from build123d import *

# Parameters (mm, degrees)
SKETCH3_W               = 76.2
SKETCH3_H               = 158.75
BOSS_EXTRUDE1_DEPTH     = 53.975
SHELL1_T                = 6
FILLET1_R               = 5.334
FILLET2_R               = 6.35
CUT_EXTRUDE1_DEPTH      = 1.2446
FILLET3_R               = 0.254
FILLET4_R               = 0.127
SKETCH7_W               = 76.2
SKETCH7_H               = 2.5
BOSS_EXTRUDE2_DEPTH     = 53.975
BOSS_EXTRUDE3_DEPTH     = 29.972
SKETCH9_R               = 3.025
CUT_EXTRUDE2_DEPTH      = 9
MIRROR2_COPY_1_DEPTH    = 29.972
MIRROR2_COPY_2_SKETCH_R = 3.025
MIRROR2_COPY_2_DEPTH    = 9
BOSS_EXTRUDE4_DEPTH     = 29.972
SKETCH11_R              = 3.025
CUT_EXTRUDE3_DEPTH      = 9
BOSS_EXTRUDE5_DEPTH     = 29.972
SKETCH13_R              = 3.025
CUT_EXTRUDE4_DEPTH      = 9
SKETCH17_R              = 9.525
SKETCH17_R_2            = 6.35
CUT_EXTRUDE6_DEPTH      = 6
SKETCH18_R              = 14.2875
SKETCH18_R_2            = 10.795
CUT_EXTRUDE7_DEPTH      = 3


with BuildPart() as part:
    # Sketch3 → Boss-Extrude1 (new body)
    with BuildSketch(Plane.XY):
        with Locations((38.1, 79.375)):
            Rectangle(SKETCH3_W, SKETCH3_H)
    extrude(amount=BOSS_EXTRUDE1_DEPTH)

    # Shell1
    shell1_openings = [part.faces().sort_by_distance(p)[0] for p in [
        (38.1, 79.375, 0),
    ]]
    offset(amount=SHELL1_T, openings=shell1_openings, kind=Kind.INTERSECTION)

    # Fillet1
    # the kernel refuses this fillet: 5.334 mm, written as the material it adds along each edge
    with BuildSketch(Plane(origin=(0, 158.75, 0), x_dir=(1, 0, 0), z_dir=(0, 0, 1)), Plane(origin=(76.2, 0, 0), x_dir=(-1, 0, 0), z_dir=(0, 0, 1)), Plane(origin=(76.2, 158.75, 0), x_dir=(0, -1, 0), z_dir=(0, 0, 1))) as fillet1_piece_1:
        with BuildLine():
            CenterArc((FILLET1_R, -FILLET1_R), FILLET1_R, 90, 90)
            Line((0, -FILLET1_R), (0, 0))
            Line((0, 0), (FILLET1_R, 0))
        make_face()
    extrude(amount=53.975)
    with BuildSketch(Plane(origin=(0, 0, 0), x_dir=(1, 0, 0), z_dir=(0, 0, 1))) as fillet1_piece_2:
        with BuildLine():
            CenterArc((FILLET1_R, FILLET1_R), FILLET1_R, 180, 90)
            Line((0, FILLET1_R), (0, 0))
            Line((0, 0), (FILLET1_R, 0))
        make_face()
    extrude(amount=53.975)

    # Fillet2
    fillet2_edges = [part.edges().sort_by_distance(p)[0] for p in [
        (-6, 164.75, 29.9875),
        (82.2, 164.75, 29.9875),
        (82.2, -6, 29.9875),
        (-6, -6, 29.9875),
    ]]
    fillet(fillet2_edges, radius=FILLET2_R)

    # Sketch6 → Cut-Extrude1 (cut)
    with BuildSketch(Plane(origin=(0, 0, 0), x_dir=(-1, 0, 0), z_dir=(0, 0, -1))):
        with BuildLine():
            Line((-5.334, 163.0327), (-70.866, 163.0327))
            ThreePointArc((-70.866, 163.0327), (-77.666033783, 160.216033783), (-80.4827, 153.416))
            Line((-80.4827, 153.416), (-80.4827, 5.334))
            ThreePointArc((-80.4827, 5.334), (-77.666033783, -1.466033783), (-70.866, -4.2827))
            Line((-70.866, -4.2827), (-5.334, -4.2827))
            ThreePointArc((-5.334, -4.2827), (1.466033783, -1.466033783), (4.2827, 5.334))
            Line((4.2827, 5.334), (4.2827, 153.416))
            ThreePointArc((4.2827, 153.416), (1.466033783, 160.216033783), (-5.334, 163.0327))
        make_face()
        with BuildLine():
            Line((-77.9173, 153.416), (-77.9173, 5.334))
            ThreePointArc((-77.9173, 5.334), (-75.852022046, 0.347977954), (-70.866, -1.7173))
            Line((-70.866, -1.7173), (-5.334, -1.7173))
            ThreePointArc((-5.334, -1.7173), (-0.347977954, 0.347977954), (1.7173, 5.334))
            Line((1.7173, 5.334), (1.7173, 153.416))
            ThreePointArc((1.7173, 153.416), (-0.347977954, 158.402022046), (-5.334, 160.4673))
            Line((-5.334, 160.4673), (-70.866, 160.4673))
            ThreePointArc((-70.866, 160.4673), (-75.852022046, 158.402022046), (-77.9173, 153.416))
        make_face(mode=Mode.SUBTRACT)
    extrude(amount=-CUT_EXTRUDE1_DEPTH, mode=Mode.SUBTRACT)

    # Fillet3
    fillet3_edges = [part.edges().sort_by_distance(p)[0] for p in [
        (-1.466033783, 160.216033783, 1.2446),
        (-4.2827, 79.375, 1.2446),
        (-1.466033783, -1.466033783, 1.2446),
        (38.1, -4.2827, 1.2446),
        (77.666033783, -1.466033783, 1.2446),
        (80.4827, 79.375, 1.2446),
        (77.666033783, 160.216033783, 1.2446),
        (38.1, 163.0327, 1.2446),
        (38.1, 160.4673, 1.2446),
        (75.852022046, 158.402022046, 1.2446),
        (77.9173, 79.375, 1.2446),
        (75.852022046, 0.347977954, 1.2446),
        (38.1, -1.7173, 1.2446),
        (0.347977954, 0.347977954, 1.2446),
        (-1.7173, 79.375, 1.2446),
        (0.347977954, 158.402022046, 1.2446),
    ]]
    fillet(fillet3_edges, radius=FILLET3_R)

    # Fillet4
    fillet4_edges = [part.edges().sort_by_distance(p)[0] for p in [
        (-1.466033783, 160.216033783, 0),
        (38.1, 163.0327, 0),
        (77.666033783, 160.216033783, 0),
        (80.4827, 79.375, 0),
        (77.666033783, -1.466033783, 0),
        (38.1, -4.2827, 0),
        (-1.466033783, -1.466033783, 0),
        (-4.2827, 79.375, 0),
        (75.852022046, 158.402022046, 0),
        (38.1, 160.4673, 0),
        (0.347977954, 158.402022046, 0),
        (-1.7173, 79.375, 0),
        (0.347977954, 0.347977954, 0),
        (38.1, -1.7173, 0),
        (75.852022046, 0.347977954, 0),
        (77.9173, 79.375, 0),
    ]]
    fillet(fillet4_edges, radius=FILLET4_R)

    # Sketch7 → Boss-Extrude2 (add)
    with BuildSketch(Plane(origin=(0, 0, 53.975), x_dir=(-1, 0, 0), z_dir=(0, 0, -1))):
        with Locations((-38.1, 36.175)):
            Rectangle(SKETCH7_W, SKETCH7_H)
    extrude(amount=BOSS_EXTRUDE2_DEPTH)

    # Sketch8 → Boss-Extrude3 (add)
    with BuildSketch(Plane(origin=(0, 0, 0), x_dir=(-1, 0, 0), z_dir=(0, 0, -1))):
        with BuildLine():
            ThreePointArc((6, 0.35), (5.516635031, -2.080039796), (4.140128061, -4.140128061))
            ThreePointArc((4.140128061, -4.140128061), (2.080039796, -5.516635031), (-0.35, -6))
            Line((-0.35, -6), (-1.778174593, -6))
            Line((-1.778174593, -6), (1.202282953, -8.980457546))
            ThreePointArc((1.202282953, -8.980457546), (8.980457546, -8.980457546), (8.980457546, -1.202282953))
            Line((8.980457546, -1.202282953), (6, 1.778174593))
            Line((6, 1.778174593), (6, 0.35))
        make_face()
    boss_extrude3 = extrude(amount=-BOSS_EXTRUDE3_DEPTH)

    # Sketch9 → Cut-Extrude2 (cut)
    with BuildSketch(Plane(origin=(0, 0, 0), x_dir=(-1, 0, 0), z_dir=(0, 0, -1))):
        with Locations((5.09137025, -5.09137025)):
            Circle(SKETCH9_R)
    cut_extrude2 = extrude(amount=-CUT_EXTRUDE2_DEPTH, mode=Mode.SUBTRACT)

    # Mirror1: Boss-Extrude3, Cut-Extrude2 across plane
    add(boss_extrude3.mirror(Plane.ZY.offset(-38.1)))
    add(cut_extrude2.mirror(Plane.ZY.offset(-38.1)), mode=Mode.SUBTRACT)

    # Mirror2: Boss-Extrude3, Cut-Extrude2 across plane
    add(boss_extrude3.mirror(Plane(origin=(0, 79.375, 0), x_dir=(0, 0, 1), z_dir=(0, -1, 0))))
    add(cut_extrude2.mirror(Plane(origin=(0, 79.375, 0), x_dir=(0, 0, 1), z_dir=(0, -1, 0))), mode=Mode.SUBTRACT)

    # Mirror2 copy 1 sketch → Mirror2 copy 1 (add)
    with BuildSketch(Plane(origin=(76.2, 158.75, 0), x_dir=(1, 0, 0), z_dir=(0, 0, -1))):
        with BuildLine():
            ThreePointArc((6, 0.35), (5.516635031, -2.080039796), (4.140128061, -4.140128061))
            ThreePointArc((4.140128061, -4.140128061), (2.080039796, -5.516635031), (-0.35, -6))
            Line((-0.35, -6), (-1.778174593, -6))
            Line((-1.778174593, -6), (1.202282953, -8.980457546))
            ThreePointArc((1.202282953, -8.980457546), (8.980457546, -8.980457546), (8.980457546, -1.202282953))
            Line((8.980457546, -1.202282953), (6, 1.778174593))
            Line((6, 1.778174593), (6, 0.35))
        make_face()
    extrude(amount=-MIRROR2_COPY_1_DEPTH)

    # Mirror2 copy 2 sketch → Mirror2 copy 2 (cut)
    with BuildSketch(Plane(origin=(76.2, 158.75, 0), x_dir=(1, 0, 0), z_dir=(0, 0, -1))):
        with Locations((5.09137025, -5.09137025)):
            Circle(MIRROR2_COPY_2_SKETCH_R)
    extrude(amount=-MIRROR2_COPY_2_DEPTH, mode=Mode.SUBTRACT)

    # Sketch10 → Boss-Extrude4 (add)
    with BuildSketch(Plane(origin=(0, 0, 0), x_dir=(-1, 0, 0), z_dir=(0, 0, -1))):
        with BuildLine():
            Line((6, 102.069), (9.4097, 102.069))
            ThreePointArc((9.4097, 102.069), (14.9097, 107.569), (9.4097, 113.069))
            Line((9.4097, 113.069), (6, 113.069))
            Line((6, 113.069), (6, 102.069))
        make_face()
        with BuildLine():
            Line((9.4097, 56.681), (6, 56.681))
            Line((6, 56.681), (6, 45.681))
            Line((6, 45.681), (9.4097, 45.681))
            ThreePointArc((9.4097, 45.681), (14.9097, 51.181), (9.4097, 56.681))
        make_face()
    boss_extrude4 = extrude(amount=-BOSS_EXTRUDE4_DEPTH)

    # Sketch11 → Cut-Extrude3 (cut)
    with BuildSketch(Plane(origin=(0, 0, 0), x_dir=(-1, 0, 0), z_dir=(0, 0, -1))):
        with Locations((9.4097, 51.181)):
            Circle(SKETCH11_R)
        with Locations((9.4097, 107.569)):
            Circle(SKETCH11_R)
    cut_extrude3 = extrude(amount=-CUT_EXTRUDE3_DEPTH, mode=Mode.SUBTRACT)

    # Mirror3: Boss-Extrude4, Cut-Extrude3 across plane
    add(boss_extrude4.mirror(Plane.ZY.offset(-38.1)))
    add(cut_extrude3.mirror(Plane.ZY.offset(-38.1)), mode=Mode.SUBTRACT)

    # Sketch12 → Boss-Extrude5 (add)
    with BuildSketch(Plane(origin=(0, 0, 0), x_dir=(-1, 0, 0), z_dir=(0, 0, -1))):
        with BuildLine():
            Line((-43.6, -6), (-43.6, -9.4097))
            ThreePointArc((-43.6, -9.4097), (-38.1, -14.9097), (-32.6, -9.4097))
            Line((-32.6, -9.4097), (-32.6, -6))
            Line((-32.6, -6), (-43.6, -6))
        make_face()
    boss_extrude5 = extrude(amount=-BOSS_EXTRUDE5_DEPTH)

    # Sketch13 → Cut-Extrude4 (cut)
    with BuildSketch(Plane(origin=(0, 0, 0), x_dir=(-1, 0, 0), z_dir=(0, 0, -1))):
        with Locations((-38.1, -9.4097)):
            Circle(SKETCH13_R)
    cut_extrude4 = extrude(amount=-CUT_EXTRUDE4_DEPTH, mode=Mode.SUBTRACT)

    # Mirror4: Boss-Extrude5, Cut-Extrude4 across plane
    add(boss_extrude5.mirror(Plane(origin=(0, 79.375, 0), x_dir=(0, 0, 1), z_dir=(0, -1, 0))))
    add(cut_extrude4.mirror(Plane(origin=(0, 79.375, 0), x_dir=(0, 0, 1), z_dir=(0, -1, 0))), mode=Mode.SUBTRACT)

    # Sketch17 → Cut-Extrude6 (cut)
    with BuildSketch(Plane.ZY.offset(6)):
        with Locations(Location((38.385, 119.975, 0), (0, 0, 270))):
            Circle(SKETCH17_R)
        with Locations(Location((38.385, 20.1295, 0), (0, 0, 270))):
            Circle(SKETCH17_R_2)
    extrude(amount=-CUT_EXTRUDE6_DEPTH, mode=Mode.SUBTRACT)

    # Sketch18 → Cut-Extrude7 (cut)
    with BuildSketch(Plane(origin=(0, 0, 0), x_dir=(0, 0, -1), z_dir=(1, 0, 0))):
        with Locations(Location((-38.385, 119.975, 0), (0, 0, 90))):
            Circle(SKETCH18_R)
        with Locations(Location((-38.385, 20.1295, 0), (0, 0, 90))):
            Circle(SKETCH18_R_2)
    extrude(amount=-CUT_EXTRUDE7_DEPTH, mode=Mode.SUBTRACT)


solid = part.part
Could you check a few things on this model? Use its own coordinates, in mm. A direction names the side the tool comes from. Coordinates: 2 decimals unless noted, no trailing zeros. Order: outer loops, then holes, each group sorted by start corner. A loop starts at its lowest first (then second) coordinate and runs counter-clockwise, first axis right, second up. Notation, with made-up numbers: (-5, 67.25) -> (0, 67.25) arc R14 ccw to (0, 88.25) -> close; hole circle Ø7 at (63.5, 29). An arc over 180 degrees is marked (long way). One line per question, with ' | ' between items.
Q1. On a 3-axis mill with a long thin cutter (end or side, diameter ignored), from which of +Z, -Z, +X, -X, +Y, -Y can I reach the whole of each face in a straight line? I mean faces 1 (the face through (-1.48, 127.66, 50.43)), 2 (the face through (88.4, 106.4, 4.4)), 3 (the face through (-6, -6, 29.972)). Say none if no direction works.
Return value:
face 1: none | face 2: -Z | face 3: +Z, -X, -Y
Q2. Imagine slicing it at A-A on z = 56. Please give me the cut outline in (x, y).
Return value:
outline: (-6, 0.35) arc R6.35 ccw to (0.35, -6) -> (75.85, -6) arc R6.35 ccw to (82.2, 0.35) -> (82.2, 158.4) arc R6.35 ccw to (75.85, 164.75) -> (0.35, 164.75) arc R6.35 ccw to (-6, 158.4) -> close
Q3. Thinking about a two-plate mould opening in X: for faces 4 (the face through (38, -6, 36)), 5 (the face through (77, 80, 0)), 6 (the face through (91.11, 51.06, 14.78)), which applies, pulls with the +X half, pulls with the -X half, needs draft (parallel to the pull), parting line crosses it, or undercut?
Return value:
face 4: undercut | face 5: needs draft | face 6: pulls with the +X half
Q4. Imagine slicing it at B-B on x = 29. Please give me the cut outline in (y, z) (3 decimals).
Return value:
outline: (-6, 0) -> (-4.41, 0) arc R0.127 ccw to (-4.283, 0.127) -> (-4.283, 0.991) arc R0.254 cw to (-4.029, 1.245) -> (-1.971, 1.245) arc R0.254 cw to (-1.717, 0.991) -> (-1.717, 0.127) arc R0.127 ccw to (-1.59, 0) -> (0, 0) -> (0, 53.975) -> (34.925, 53.975) -> (34.925, 0) -> (37.425, 0) -> (37.425, 53.975) -> (158.75, 53.975) -> (158.75, 0) -> (160.34, 0) arc R0.127 ccw to (160.467, 0.127) -> (160.467, 0.991) arc R0.254 cw to (160.721, 1.245) -> (162.779, 1.245) arc R0.254 cw to (163.033, 0.991) -> (163.033, 0.127) arc R0.127 ccw to (163.16, 0) -> (164.75, 0) -> (164.75, 59.975) -> (-6, 59.975) -> close
Q5. If I drill on L1, parallel to Y at x = 31, z = 47.5 (3 decimals); L2, parallel to Y at x = 3.5, z = 12.5 (3 decimals); L3, parallel to X at y = 112, z = 51, over which ranges is the centre line in solid material (lowest first)?
Return value:
L1: -6 to 0, 34.925 to 37.425, 158.75 to 164.75 | L2: -6 to 0.325, 34.925 to 37.425, 158.425 to 164.75 | L3: -6 to 0, 76.2 to 82.2
Q6. I'm going to push flat-ended pins straight in: P1, Ø4, axis at x = 77, z = 43, coming from the +Y side; P2, Ø5, axis at y = 81, z = 20, coming from the +X side; P3, Ø12, axis at x = 70.5, z = 49, coming from the -Y side. Where does each tip first touch, or does it pass through?
Return value:
P1: y = 164.75 | P2: x = 82.2 | P3: y = -6
